Could you check a few things on this drawing? It's one solid part, dimensions in mm from its lowest x, y, z. A direction names the side the tool comes from. Give positions to 0.01 mm unless a question says otherwise; leave off trailing zeros. Write each loop counter-clockwise with the first axis right and the second up, starting at its lowest first coordinate (ties: lowest second). Pieces come first, ordered by that corner, then holes. Notation, with made-up numbers: M 38.25,7.5 L 88.25,7.5 A11 cw 88.25,26.5 Z; hole C 21.25,76.25 d4. An arc over 180 degrees is marked long. Answer as CSV lines item,"result". Start each with the question number.
Q1. Suppose I cut it at A-A (y = 8). Write out the boundary of the cut face in (x, z).
Q2. On a 3-axis mill with a long thin cutter (end or side, diameter ignored), from which of +Z, -Z, +X, -X, +Y, -Y can I reach the whole of each face in a straight line? I mean the marked faces 1 and 2. Say none if no direction works.
Q3. Thinking about a two-plate mould opening in Y: for the marked faces 3, 4, 5 and 6, which applies, +Y half, -Y half, draft (parallel to the pull), parting line (faces both ways), or undercut?
Q4. Suppose I cut it at C-C (z = 2.5). Write out the boundary of the cut face in (x, y), then the cut area to 3 significant figures.
Q5. If I drill on line 1 along Y through (x, z) = (5, 0.5); line 2 along X through (y, z) = (5, 0.25); line 3 along X through (y, z) = (2, 0.8), over which ranges is the centre line in solid material (lowest first)?
Q6. Suppose I cut it at B-B (x = 7). Write out the boundary of the cut face in (y, z).
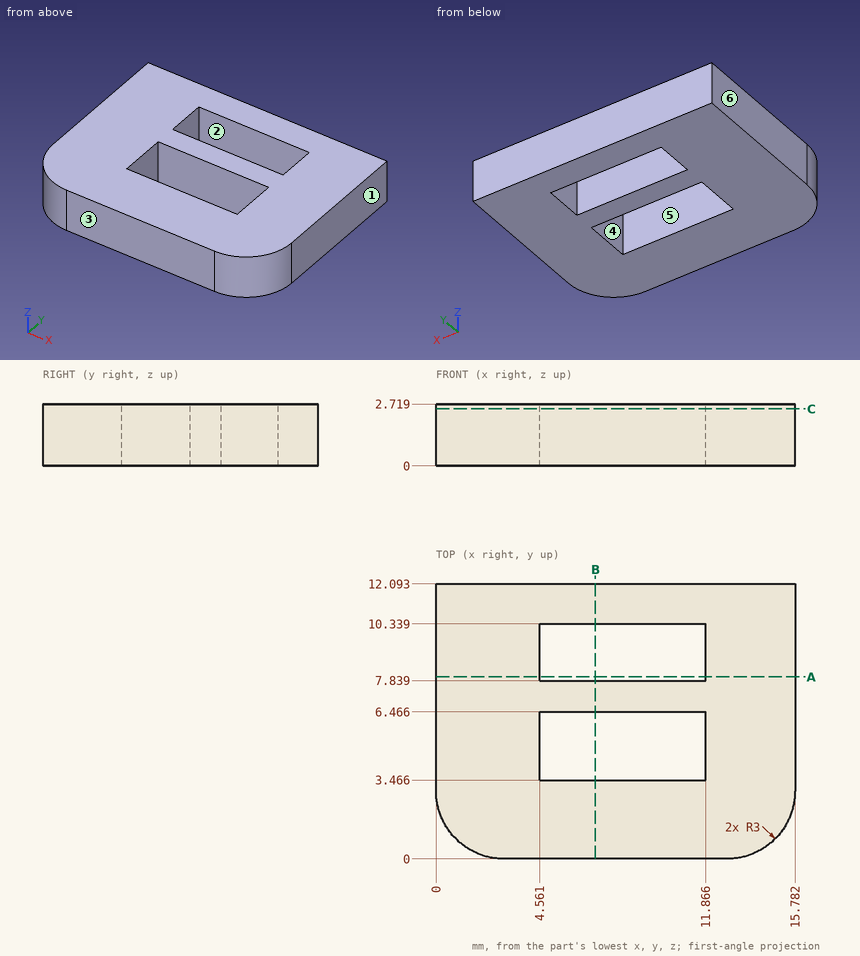
Resolved:
1,outline,"M 0,0 L 4.56,0 L 4.56,2.72 L 0,2.72 Z; M 11.87,0 L 15.78,0 L 15.78,2.72 L 11.87,2.72 Z"
2,face 1,"+Z, -Z, +X, +Y, -Y"
2,face 2,"+Z, -Z"
3,face 3,"-Y half"
3,face 4,"undercut"
3,face 5,"undercut"
3,face 6,"draft"
4,outline,"M 0,3 A3 ccw 3,0 L 12.78,0 A3 ccw 15.78,3 L 15.78,12.09 L 0,12.09 Z; hole M 4.56,3.47 L 11.87,3.47 L 11.87,6.47 L 4.56,6.47 Z; hole M 4.56,7.84 L 11.87,7.84 L 11.87,10.34 L 4.56,10.34 Z"
4,area,"147 mm^2"
5,line 1,"0 to 3.47, 6.47 to 7.84, 10.34 to 12.09"
5,line 2,"0 to 4.56, 11.87 to 15.78"
5,line 3,"0.17 to 15.61"
6,outline,"M 0,0 L 3.47,0 L 3.47,2.72 L 0,2.72 Z; M 6.47,0 L 7.84,0 L 7.84,2.72 L 6.47,2.72 Z; M 10.34,0 L 12.09,0 L 12.09,2.72 L 10.34,2.72 Z"
